Here's the drawing with two shaded views (mm, measured from the low corner). I have some questions. A direction names the side the tool comes from. Give positions to 0.01 mm unless a question says otherwise; leave off trailing zeros. Loops run counter-clockwise (first coordinate to the right, second up) from the corner with the lowest first, then second, coordinate; pieces in that order, holes last.
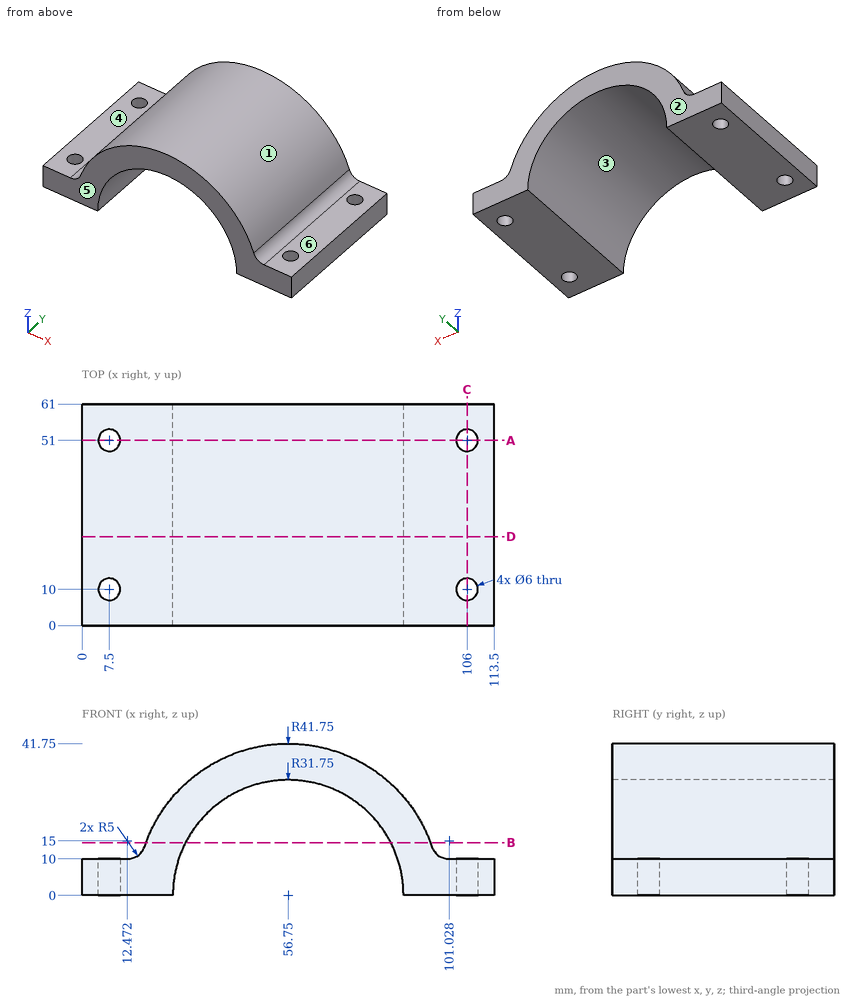
(1) Will these pins go through, and if not, where does the flat tip stop? P1, Ø8, axis at y = 47.5, z = 17, coming from the -X side; P2, Ø1, axis at y = 28.5, z = 21, coming from the +X side; P3, Ø13.5, axis at x = 108.5, y = 32.5, coming from the +Z side; P4, Ø5, axis at x = 7.5, y = 51, coming from the +Z side.
Returned:
P1: stops at x = 17.05
P2: stops at x = 93.12
P3: stops at z = 10
P4: passes through
(2) Suppose I cut it at C-C on x = 106. List the corners of the cut face in (y, z) for me, plus the area to 3 significant figures.
Returned:
outline: (0, 0) - (7, 0) - (7, 10) - (0, 10) - close; (13, 0) - (48, 0) - (48, 10) - (13, 10) - close; (54, 0) - (61, 0) - (61, 10) - (54, 10) - close
area: 490 mm2
(3) Thinking about a two-plate mould opening in X: for the marked faces 1, 2 and 3, which applies, pulls with the +X half, pulls with the -X half, needs draft (parallel to the pull), parting line crosses it, or undercut?
Returned:
face 1: parting line crosses it
face 2: needs draft
face 3: undercut
(4) Suppose I cut it at A-A on y = 51. List the corners of the cut face in (x, z) for me.
Returned:
outline: (0, 0) - (4.5, 0) - (4.5, 10) - (0, 10) - close; (10.5, 0) - (25, 0) arc R31.75 cw to (88.5, 0) - (103, 0) - (103, 10) - (101.03, 10) arc R5 cw to (96.29, 13.4) arc R41.75 ccw to (17.21, 13.4) arc R5 cw to (12.47, 10) - (10.5, 10) - close; (109, 0) - (113.5, 0) - (113.5, 10) - (109, 10) - close
(5) Suppose I cut it at B-B on z = 14.5. List the corners of the cut face in (x, y) for me, plus the area to 3 significant figures.
Returned:
outline: (17.6, 0) - (28.5, 0) - (28.5, 61) - (17.6, 61) - close; (85, 0) - (95.9, 0) - (95.9, 61) - (85, 61) - close
area: 1,330 mm2
(6) Which directions (+Z, -Z, +X, -X, +Y, -Y) give clear straight access to the entire face, cutting with the end or side of a thin tool? Please do the marked faces 4, 5 and 6.
Returned:
face 4: +Z, -X, +Y, -Y
face 5: +Z, -Z, +X, -X, -Y
face 6: +Z, +X, +Y, -Y
(7) Please list where these lines run through material, in increasing order: probe 1 along Y at (x, z) = (106, 6.25); probe 2 along X at (y, z) = (12, 5) (1 decimal); probe 3 along X at (y, z) = (12, 14.5) (1 decimal).
Returned:
probe 1: y = 0 to 7, 13 to 48, 54 to 61
probe 2: x = 0 to 5.3, 9.7 to 25.4, 88.1 to 103.8, 108.2 to 113.5
probe 3: x = 17.6 to 28.5, 85 to 95.9
(8) Suppose I cut it at D-D on y = 24.5. List the corners of the cut face in (x, z) for me.
Returned:
outline: (0, 0) - (25, 0) arc R31.75 cw to (88.5, 0) - (113.5, 0) - (113.5, 10) - (101.03, 10) arc R5 cw to (96.29, 13.4) arc R41.75 ccw to (17.21, 13.4) arc R5 cw to (12.47, 10) - (0, 10) - close
